Here's how the part is built. I have some questions about the finished solid (model axes, mm). Coordinates: 2 decimals unless noted, no trailing zeros. Write each loop counter-clockwise with the first axis right and the second up, starting at its lowest first coordinate (ties: lowest second). Pieces come first, ordered by that corner, then holes. Notation, with made-up numbers: (59, 37.5) -> (85, 37.5) arc R23 ccw to (85, 76.5) -> close; hole circle Ø4 at (-22, 88.5). An arc over 180 degrees is marked (long way). Put each result on its own line as item: value. Start each with the question number.
Item 1: For pin 1 (1.5 mm diameter, centred on x = -16.5, y = 0.5, fed in from -Z); pin 2 (1.9 mm diameter, centred on x = -16.26, z = -16.26, fed in from +Y); pin 3 (4 mm diameter, centred on x = -23, z = 0, fed in from +Y); pin 4 (3 mm diameter, centred on x = 16.26, z = -16.26, fed in from +Y), each with a flat end and sliding along its axis, tell me the tip position at first contact or that it passes through.
Item 2: I want a section at B-B, the plane y = 1.4. State how many separate pieces and enclosed holes the cut face has, then the cut area to 3 significant figures.
Item 3: I want a section at A-A, the plane x = 0. List the corners of the cut face in (y, z) for me.
Item 4: I need wall thicknesses on line 1 (X direction, y = 1.65, z = 0); line 2 (Z direction, x = 17, y = 1.55); line 3 (X direction, y = 2.35, z = -1). Which ranges of each line are inside material? Lowest first, please. Write a range as [from, to].
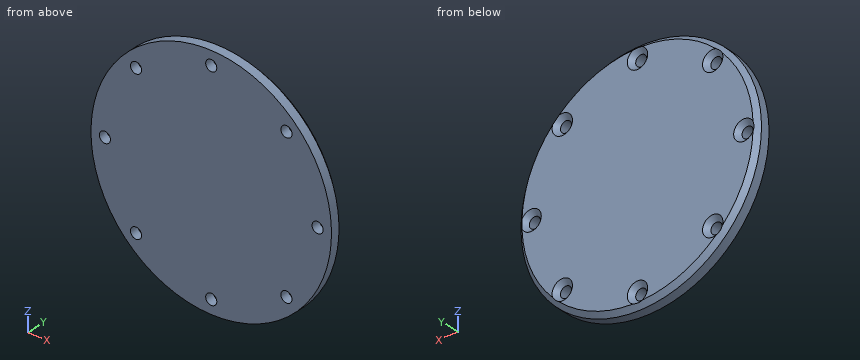
from build123d import *

# Parameters (mm, degrees)
HOLE_WIZARD_M21_D           = 2.4
HOLE_WIZARD_M21_CSINK_D     = 4.4
HOLE_WIZARD_M21_CSINK_ANGLE = 90
PATTERN_CIRCULAR_1_COUNT    = 8


with BuildPart() as part:
    # Эскиз1 → Повернуть1 (revolve)
    with BuildSketch(Plane.XY, mode=Mode.PRIVATE) as revolve_1_sk:
        Polygon((0, 0), (26, 0), (26, 2), (25, 3), (0, 3), align=None)
    revolve(revolve_1_sk.sketch.rotate(Axis((0, 0, 0), (0, 1, 0)), 90), axis=Axis((0, 0, 0), (0, 1, 0)))

    # Зенковка для винта с потайной головкой M21 (through all)
    with Locations(Plane(origin=(0, 3, 0), x_dir=(1, 0, 0), z_dir=(0, 1, 0))):
        with Locations((16.263455967, 16.263455967)):
            hole_wizard_m21 = CounterSinkHole(HOLE_WIZARD_M21_D / 2, HOLE_WIZARD_M21_CSINK_D / 2, counter_sink_angle=HOLE_WIZARD_M21_CSINK_ANGLE)

    # Круговой массив1: Зенковка для винта с потайной головкой M21 ×8 about axis
    pattern_circular_1_axis = Axis((0, 0, 0), (0, 1, 0))
    for i in range(1, PATTERN_CIRCULAR_1_COUNT):
        add(hole_wizard_m21.rotate(pattern_circular_1_axis, i * 360 / PATTERN_CIRCULAR_1_COUNT), mode=Mode.SUBTRACT)


solid = part.part
Calculated:
1. pin 1: stops at z = -20.69
1. pin 2: passes through
1. pin 3: stops at y = 2.8
1. pin 4: stops at y = 2.3
2. separate pieces: 1
2. enclosed holes: 8
2. area: 2,090 mm2
3. outline: (0, -26) -> (2, -26) -> (2.9, -25.1) -> (2, -24.2) -> (0, -24.2) -> close; (0, -21.8) -> (2, -21.8) -> (3, -20.8) -> (3, 20.8) -> (2, 21.8) -> (0, 21.8) -> close; (0, 24.2) -> (2, 24.2) -> (2.9, 25.1) -> (2, 26) -> (0, 26) -> close
4. line 1: x = [-26, -24.2], [-21.8, 21.8], [24.2, 26]
4. line 2: z = [-19.67, -17.21], [-15.32, 15.32], [17.21, 19.67]
4. line 3: x = [-25.63, -24.18], [-21.82, 21.82], [24.18, 25.63]
